```python
from build123d import *

# Parameters (mm, degrees)
BOSS_EXTRUDE1_DEPTH = 150
BOSS_EXTRUDE2_START = -20
BOSS_EXTRUDE2_DEPTH = 20
SKETCH3_R           = 5
CUT_EXTRUDE1_DEPTH  = 20
CUT_EXTRUDE2_DEPTH  = 10


with BuildPart() as part:
    # Sketch1 → Boss-Extrude1 (new body)
    with BuildSketch(Plane.XY):
        with BuildLine():
            Line((30, 0), (27.5, 0))
            ThreePointArc((27.5, 0), (0, -27.5), (-27.5, 0))
            Line((-27.5, 0), (-30, 0))
            ThreePointArc((-30, 0), (0, -30), (30, 0))
        make_face()
    extrude(amount=BOSS_EXTRUDE1_DEPTH)

    # Sketch2 → Boss-Extrude2 (add)
    with BuildSketch(Plane.XY.offset(150).offset(BOSS_EXTRUDE2_START)):
        with BuildLine():
            Line((0, -45.496190277), (0, -30))
            ThreePointArc((0, -30), (-2.508787808, -29.894915684), (-5, -29.580398915))
            Line((-5, -29.580398915), (-5, -48))
            Line((-5, -48), (0, -48))
            Line((0, -48), (0, -45.496190277))
        make_face()
        with BuildLine():
            ThreePointArc((5, -29.580398915), (2.508787808, -29.894915684), (0, -30))
            Line((0, -30), (0, -45.496190277))
            Line((0, -45.496190277), (0, -48))
            Line((0, -48), (5, -48))
            Line((5, -48), (5, -29.580398915))
        make_face()
    extrude(amount=BOSS_EXTRUDE2_DEPTH)

    # Sketch3 → Cut-Extrude1 (cut)
    with BuildSketch(Plane(origin=(5, 0, 0), x_dir=(0, 0, -1), z_dir=(1, 0, 0))):
        with Locations(Location((-140, -39.580398915, 0), (0, 0, 90))):
            Circle(SKETCH3_R)
    extrude(amount=-CUT_EXTRUDE1_DEPTH, mode=Mode.SUBTRACT)

    # Sketch4 → Cut-Extrude2 (cut)
    with BuildSketch(Plane(origin=(5, 0, 0), x_dir=(0, 0, -1), z_dir=(1, 0, 0))):
        with BuildLine():
            ThreePointArc((-134, -39.580398915), (-140, -45.580398915), (-146, -39.580398915))
            Line((-146, -39.580398915), (-146, -29.580398915))
            Line((-146, -29.580398915), (-150, -29.580398915))
            Line((-150, -29.580398915), (-150, -48))
            Line((-150, -48), (-130, -48))
            Line((-130, -48), (-130, -29.580398915))
            Line((-130, -29.580398915), (-134, -29.580398915))
            Line((-134, -29.580398915), (-134, -39.580398915))
        make_face()
    extrude(amount=-CUT_EXTRUDE2_DEPTH, mode=Mode.SUBTRACT)


solid = part.part
```
Part model, mm, in its own coordinate system. A direction names the side the tool comes from. Round coordinates to 2 decimals unless told otherwise and drop trailing zeros. Write each loop counter-clockwise with the first axis right and the second up, starting at its lowest first coordinate (ties: lowest second). Pieces come first, ordered by that corner, then holes.
Item 1: Which spindle directions (+Z, -Z, +X, -X, +Y, -Y) get a long thin tool onto all of the face, cutting with end or side? Do faces 4 (the flat face through (-5, -34, 140)), 5 (the flat face through (0, -29.58, 148)), 6 (the flat face through (0, -29.58, 132)), 7 (the flat face through (5, -34, 140)). Say none if no direction does.
Results:
face 4: +Z, -Z, -X, -Y
face 5: +Z, +X, -X, -Y
face 6: +X, -X, -Y
face 7: +Z, -Z, +X, -Y
Item 2: Cut at A-A, the plane z = 140. Give the cut face in (x, y).
Results:
outline: (-30, 0) arc R30 ccw to (-5, -29.58) - (-5, -34.58) - (5, -34.58) - (5, -29.58) arc R30 ccw to (30, 0) - (27.5, 0) arc R27.5 cw to (-27.5, 0) - close; (-5, -45.58) - (5, -45.58) - (5, -44.58) - (-5, -44.58) - close
Item 3: Two-plate mould, pull along X, no slides. Class faces 1 (the cylindrical face through (-0.66, -29.993, 73.95)), 2 (the flat face through (0, -35, 134)), 3 (the cylindrical face through (0.605, -27.493, 73.95)): +X half, -X half, draft (parallel to the pull), parting line (faces both ways), or undercut.
Results:
face 1: parting line
face 2: draft
face 3: undercut
Item 4: Drop flat-ended pins along their axis: pin 1 Ø1 at (y, z) = (-24, 25.5) entering from +X; pin 2 Ø5 at (x, y) = (0.5, -37) entering from -Z; pin 3 Ø2 at (x, z) = (6.5, 86.5) entering from +Y. Give the stop position or say it passes through.
Results:
pin 1: stops at x = 18.65
pin 2: stops at z = 134
pin 3: stops at y = -26.46
Item 5: Cut at B-B, the plane y = -13. Give the cut face in (x, z).
Results:
outline: (-27.04, 0) - (-24.23, 0) - (-24.23, 150) - (-27.04, 150) - close; (24.23, 0) - (27.04, 0) - (27.04, 150) - (24.23, 150) - close
Item 6: Cut at D-D, the plane z = 64. Give the cut face in (x, y), plus the area to 3 significant figures.
Results:
outline: (-30, 0) arc R30 ccw to (30, 0) - (27.5, 0) arc R27.5 cw to (-27.5, 0) - close
area: 226 mm2
Item 7: Cut at C-C, the plane x = 0. Give the cut face in (y, z).
Results:
outline: (-39.58, 134) - (-29.58, 134) - (-29.58, 130) - (-30, 130) - (-30, 0) - (-27.5, 0) - (-27.5, 150) - (-29.58, 150) - (-29.58, 146) - (-39.58, 146) arc R6 ccw to start; hole circle Ø10 at (-39.58, 140)
Item 8: Probe L1, parallel to X at y = -15, z = 60; L2, parallel to X at y = -13, z = 62.5; L3, parallel to Y at x = 18, z = 63.5. List the from-to ranges inside material, lowest first.
Results:
L1: x = -25.98 to -23.05, 23.05 to 25.98
L2: x = -27.04 to -24.23, 24.23 to 27.04
L3: y = -24 to -20.79
